Check sheet for the drawn part. Datum: minimum x, y, z corner. Units: mm. Coordinates: 2 decimals unless noted, no trailing zeros. Write each loop counter-clockwise with the first axis right and the second up, starting at its lowest first coordinate (ties: lowest second). Pieces come first, ordered by that corner, then holes. Notation, with made-up numbers: (-1, -16.5) -> (9, -16.5) arc R26 cw to (9, 3.5) -> close; hole circle Ø2 at (48, 47.25). An arc over 180 degrees is marked (long way). Write item = value, one per line. Start each with the question number.
(1) Mould release check, pull along X, two halves, no side actions. Record for the marked faces 1, 2 and 3: released by +X, released by -X, zero draft, split by the parting line, or undercut.
(2) Section check C-C (z = 1.5). Record the cut outline in (x, y) (3 decimals).
(3) Gauge pin test, flat ends, axial feed: pin 1 Ø3 at (x, z) = (33.5, 4.5) entering from +Y; pin 2 Ø1.5 at (x, z) = (23, 5) entering from +Y; pin 3 Ø4 at (y, z) = (89, 6) entering from -X. Record the tip position at first contact, or that the pin passes through.
(4) Section check A-A (x = 54.5). Record the cut outline in (y, z), plus the area to 3 significant figures.
(5) Section check D-D (y = 9). Record the cut outline in (x, z).
(6) Material ranges on probe 1 along X at (y, z) = (82, 9.5); probe 2 along X at (y, z) = (81.5, 1); probe 3 along Y at (x, z) = (58, 8), recorded low to high. Write a range as [from, to].
(7) Section check B-B (y = 57.5). Record the cut outline in (x, z), plus the area to 3 significant figures.
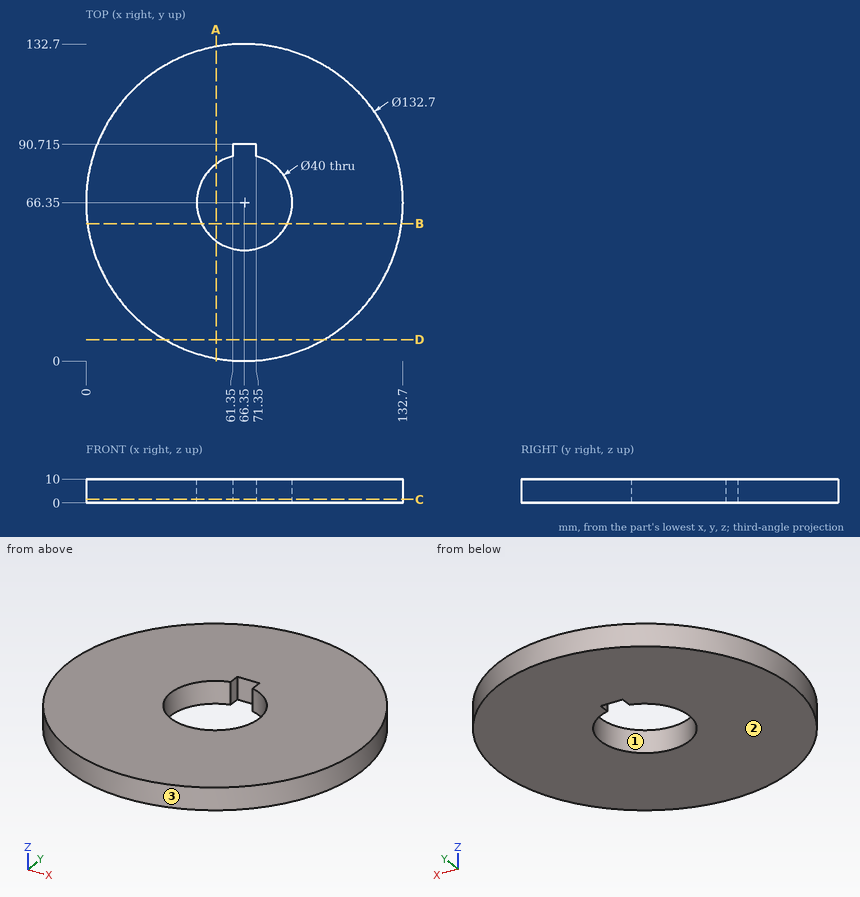
Response:
q1.face_1 = undercut
q1.face_2 = zero draft
q1.face_3 = split by the parting line
q2.outline = circle Ø132.7 at (66.35, 66.35); hole (61.35, 85.715) arc R20 ccw (long way) to (71.35, 85.715) -> (71.35, 90.715) -> (61.35, 90.715) -> close
q3.pin_1 = 124.83
q3.pin_2 = 117.22
q3.pin_3 = 3.3
q4.outline = (1.07, 0) -> (50.24, 0) -> (50.24, 10) -> (1.07, 10) -> close; (82.46, 0) -> (131.63, 0) -> (131.63, 10) -> (82.46, 10) -> close
q4.area = 983 mm2
q5.outline = (32.98, 0) -> (99.72, 0) -> (99.72, 10) -> (32.98, 10) -> close
q6.probe_1 = [1.87, 53.9], [78.8, 130.83]
q6.probe_2 = [1.75, 53.29], [79.41, 130.95]
q6.probe_3 = [0.53, 48.18], [84.52, 132.17]
q7.outline = (0.59, 0) -> (48.41, 0) -> (48.41, 10) -> (0.59, 10) -> close; (84.29, 0) -> (132.11, 0) -> (132.11, 10) -> (84.29, 10) -> close
q7.area = 956 mm2
